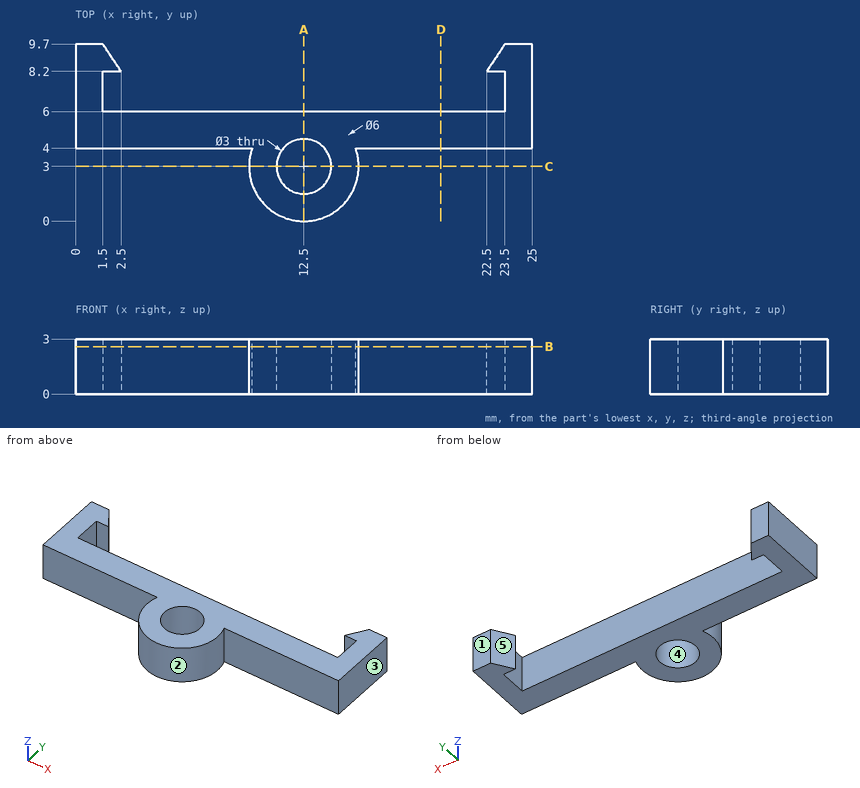
Study the drawing (mm; zero at the part's minimum x, y, z) and answer. A direction names the side the tool comes from. Give positions to 0.01 mm unless a question says otherwise; leave off trailing zeros. Loops run counter-clockwise (first coordinate to the right, second up) from the corner with the lowest first, then second, coordinate; pieces in that order, holes last. Notation, with made-up numbers: (66, 5.25) - (78, 5.25) arc R20 cw to (78, 21.25) - close; hole circle Ø6 at (43.25, 16.5). An arc over 180 degrees is marked (long way). Answer in a Markdown table with one row per item. Add a question column.
Q1. Determine the mould class of the marked faces 1, 2 and 3 for opening direction Y: released by +Y, released by -Y, zero draft, split by the parting line, or undercut.
Q2. The part is cut by section B-B (z = 2.6). Determine the outline of the cut face in (x, y), and give its area (3 significant figures).
Q3. The part is cut by section D-D (x = 20). Determine the outline of the cut face in (y, z), and give its area (3 significant figures).
Q4. The part is cut by section A-A (x = 12.5). Determine the outline of the cut face in (y, z), and give its area (3 significant figures).
Q5. A tool of negligible diameter and unlimited length cuts with its end or side. For the marked faces 4 and 5, from which of +Z, -Z, +X, -X, +Y, -Y can it reach the whole face along a straight path? Write none if from no direction.
Q6. Each of these flat-tipped pins is pushed along its axis until it touches: P1, Ø1.1, axis at x = 23, z = 1.5, coming from the -Y side; P2, Ø0.9, axis at x = 16, z = 1.5, coming from the +Y side. Where does it stop, or does it pass through?
Q7. Consider line 1 along Y through (x, z) = (12.5, 1.5); line 2 along X through (y, z) = (6.25, 1); line 3 along Y through (x, z) = (4, 1.7). Determine where each line is inside the solid, lowest interval first.
Q8. The part is cut by section C-C (y = 3). Determine the outline of the cut face in (x, z), and give its area (3 significant figures).
Solution:
| question | item | result |
|---|---|---|
| 1 | face 1 | released by +Y |
| 1 | face 2 | undercut |
| 1 | face 3 | zero draft |
| 2 | outline | (0, 4) - (9.67, 4) arc R3 ccw (long way) to (15.33, 4) - (25, 4) - (25, 9.7) - (23.5, 9.7) - (22.5, 8.2) - (23.5, 8.2) - (23.5, 6) - (1.5, 6) - (1.5, 8.2) - (2.5, 8.2) - (1.5, 9.7) - (0, 9.7) - close; hole circle Ø3 at (12.5, 3) |
| 2 | area | 75.6 mm² |
| 3 | outline | (4, 0) - (6, 0) - (6, 3) - (4, 3) - close |
| 3 | area | 6.00 mm² |
| 4 | outline | (0, 0) - (1.5, 0) - (1.5, 3) - (0, 3) - close; (4.5, 0) - (6, 0) - (6, 3) - (4.5, 3) - close |
| 4 | area | 9.00 mm² |
| 5 | face 4 | +Z, -Z |
| 5 | face 5 | +Z, -Z, +Y |
| 6 | P1 | stops at y = 4 |
| 6 | P2 | stops at y = 6 |
| 7 | line 1 | y = 0 to 1.5, 4.5 to 6 |
| 7 | line 2 | x = 0 to 1.5, 23.5 to 25 |
| 7 | line 3 | y = 4 to 6 |
| 8 | outline | (9.5, 0) - (11, 0) - (11, 3) - (9.5, 3) - close; (14, 0) - (15.5, 0) - (15.5, 3) - (14, 3) - close |
| 8 | area | 9.00 mm² |
